from build123d import *

# Parameters (mm, degrees)
F1_DEPTH    = 25.4
F2_R        = 5.08
F3_T        = -2.54
F4_T1_DEPTH = 50.8
F4_T3_DEPTH = 39.0278032796
F4_T5_DEPTH = 51.0230548821
F4_T7_DEPTH = 37.4321438382
F6_DEPTH    = 105.664


# Not quite as in the source:
# - a fillet or chamfer that OpenCascade refuses, or shapes differently, is made with other operations: its cross-section is extruded or revolved along the edge and cut away or added


with BuildPart() as f1:
    # F0 (on Top) → F1 (new body)
    with BuildSketch(Plane.XY):
        Polygon((-0.8999820115, 8.1055370808), (-10.6966300514, 1.1199682045), (6.2161790492, -17.8304114309), (17.312023155, -9.9184416504), align=None)
    extrude(amount=F1_DEPTH)

    # F2
    f2_edges = [f1.edges().sort_by_distance(p)[0] for p in [
        (8.206021, -0.906452, 25.4),
        (11.764101, -13.874427, 25.4),
        (-2.240226, -8.355222, 25.4),
        (-5.798306, 4.612753, 25.4),
    ]]
    fillet(f2_edges, radius=F2_R)

    # F3
    f3_openings = [f1.faces().sort_by_distance(p)[0] for p in [
        (3.164917, -4.822441, 0),
    ]]
    offset(amount=F3_T, openings=f3_openings)

    # F4: fillet of radius 5.08 on 4 edges, made by hand

    # F4_s2 → F4_t1 (cut)
    with BuildSketch(Plane(origin=(-13.7553254463, 15.4124981643, 0), x_dir=(0, 0, 1), z_dir=(0.665858626, -0.7460779384, 0))):
        with BuildLine():
            ThreePointArc((5.08, 7.2347792067), (1.4878975516, 5.7468816552), (0, 2.1547792067))
            Line((0, 2.1547792067), (0, 7.2347792067))
            Line((0, 7.2347792067), (5.08, 7.2347792067))
        make_face()
    extrude(amount=F4_T1_DEPTH, mode=Mode.SUBTRACT)

    # F4_s4 → F4_t3 (cut)
    with BuildSketch(Plane(origin=(-14.6481007776, -10.4449314165, 0), x_dir=(0, 0, 1), z_dir=(0.8142063602, 0.5805755791, 0))):
        with BuildLine():
            ThreePointArc((5.08, 18.1265961431), (1.4878975516, 16.6386985916), (0, 13.0465961431))
            Line((0, 13.0465961431), (0, 18.1265961431))
            Line((0, 18.1265961431), (5.08, 18.1265961431))
        make_face()
    extrude(amount=F4_T3_DEPTH, mode=Mode.SUBTRACT)

    # F4_s6 → F4_t5 (cut)
    with BuildSketch(Plane(origin=(22.7315266592, -22.496839271, 0), x_dir=(0, 0, 1), z_dir=(-0.7107663489, 0.7034281749, 0))):
        with BuildLine():
            ThreePointArc((5.08, 5.1280702931), (1.4878975516, 3.6401727415), (0, 0.0480702931))
            Line((0, 0.0480702931), (0, 5.1280702931))
            Line((0, 5.1280702931), (5.08, 5.1280702931))
        make_face()
    extrude(amount=F4_T5_DEPTH, mode=Mode.SUBTRACT)

    # F4_s8 → F4_t7 (cut)
    with BuildSketch(Plane(origin=(13.575348792, 9.6799980584, 0), x_dir=(0, 0, 1), z_dir=(-0.8142063602, -0.5805755791, 0))):
        with BuildLine():
            ThreePointArc((5.08, 7.1220874215), (1.4878975516, 5.6341898699), (0, 2.0420874215))
            Line((0, 2.0420874215), (0, 7.1220874215))
            Line((0, 7.1220874215), (5.08, 7.1220874215))
        make_face()
    extrude(amount=F4_T7_DEPTH, mode=Mode.SUBTRACT)

    # F5 (on face) → F6 (cut)
    with BuildSketch(Plane(origin=(10.5238590523, -14.7587898685, 0), x_dir=(0.8142063602, 0.5805755791, 0), z_dir=(0.5805755791, -0.8142063602, 0))):
        with BuildLine():
            Line((8.3371543562, 6.3802872405), (8.3371543562, 16.698849146))
            ThreePointArc((8.3371543562, 16.698849146), (2.6890388134, 11.5395681933), (8.3371543562, 6.3802872405))
        make_face()
        with BuildLine():
            ThreePointArc((8.3371543562, 6.3802872405), (11.6943719949, 8.0457081644), (13.0499085036, 11.5395681933))
            ThreePointArc((13.0499085036, 11.5395681933), (11.6943719949, 15.0334282221), (8.3371543562, 16.698849146))
            Line((8.3371543562, 16.698849146), (8.3371543562, 6.3802872405))
        make_face()
    extrude(amount=-F6_DEPTH, mode=Mode.SUBTRACT)


solid = f1.part
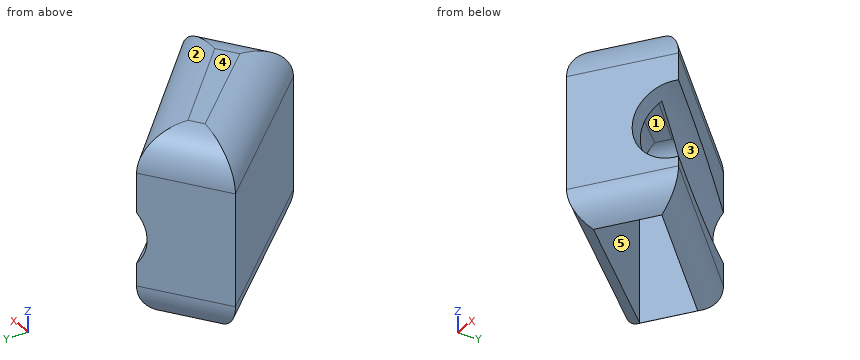
Input: part model. Units: mm. Frame: model coordinates. Face numbers are marked on the shaded views. A direction names the side the tool comes from. Give positions to 0.01 mm unless a question says otherwise; leave off trailing zeros. Write each loop counter-clockwise with the first axis right and the second up, starting at its lowest first coordinate (ties: lowest second). Pieces come first, ordered by that corner, then holes. Notation, with made-up numbers: M 24,45.25 L 65,45.25 A32 cw 65,81.25 Z; hole C 20,-33 d4. An arc over 180 degrees is marked long. Use one line per item in the form item = value.
1. Cut plane A-A on z = 18.5. Return loops of the section in (x, y).
Outcome:
outline = M -10.7,1.12 L 6.22,-17.83 L 17.31,-9.92 L -0.9,8.11 Z; hole M -6.91,0.7 L 6.6,-14.44 L 13.38,-9.6 L -1.17,4.8 Z
2. Reachability of the marked faces 1 and 2 from +Z, -Z, +X, -X, +Y, -Y: full face, straight path, thin tool, end or side. Return the list, or none.
Outcome:
face_1 = -Z
face_2 = +Z, +X, +Y
3. Cut plane C-C on z = 22. Return loops of the section in (x, y), and give its area (3 significant figures).
Outcome:
outline = M -10.27,1.07 L 6.26,-17.45 L 16.87,-9.88 L -0.93,7.73 Z; hole M -5.97,0.59 L 6.69,-13.59 L 12.4,-9.52 L -1.23,3.97 Z
area = 181 mm²
4. First-contact query: P1, Ø1, axis at y = 4, z = 19.5, coming from the +X side; P2, Ø1, axis at x = 3.5, z = 3.5, coming from the +Y side; P3, Ø3, axis at x = 2, z = 7.5, coming from the +Y side; P4, Ø12, axis at y = -5.5, z = 8.5, coming from the +X side. Flat tips, straight axial feed; report the tip coordinate or a pass-through.
Outcome:
P1 = 3.75
P2 = 3.94
P3 = 6.72
P4 = 17.31
5. Mould query, pull axis Z, two halves, no side actions, for the marked faces 3, 4 and 5. Classes: released by +Z, released by -Z, zero draft, split by the parting line, or undercut.
Outcome:
face_3 = undercut
face_4 = released by +Z
face_5 = zero draft
6. Cut plane B-B on z = 14. Return loops of the section in (x, y).
Outcome:
outline = M -10.7,1.12 L 6.22,-17.83 L 13.22,-12.84 L 11.74,-10.77 L 6.6,-14.44 L -6.91,0.7 L -1.17,4.8 L 4.99,-1.3 L -1.44,7.72 Z
7. Cut plane D-D on z = 11. Return loops of the section in (x, y), and give its area (3 significant figures).
Outcome:
outline = M -10.7,1.12 L 6.22,-17.83 L 12.74,-13.18 L 11.26,-11.11 L 6.6,-14.44 L -6.91,0.7 L -1.17,4.8 L 2.52,1.15 L -1.92,7.38 Z
area = 102 mm²
8. Ray query, L1, parallel to X at y = -10.5, z = 15.25; L2, parallel to Y at x = 3, z = 18.5; L3, parallel to Y at x = 7.75, z = 6. Return the intervals inside material, ascending.
Outcome:
L1 = -0.33 to 3.08, 12.12 to 12.71
L2 = -14.23 to -10.41, 0.67 to 4.25
L3 = -16.74 to -13.62, -4.03 to -0.46
